```python
from build123d import *

# Parameters (mm, degrees)
F0_W     = 114.3
F0_H     = 76.2
F1_DEPTH = 3.175
F2_W     = 1.881292
F2_H     = 62.23
F3_DEPTH = 6.35


with BuildPart() as f1:
    # F0 (on Front) → F1 (new body)
    with BuildSketch(Plane.XZ):
        Rectangle(F0_W, F0_H)
    extrude(amount=-F1_DEPTH)

    # F2 (on face) → F3 (join)
    with BuildSketch(Plane.XZ):
        with Locations((-49.605354, 0)):
            Rectangle(F2_W, F2_H)
        with Locations((-38.683354, 0)):
            Rectangle(F2_W, F2_H)
        with Locations((-27.761354, 0)):
            Rectangle(F2_W, F2_H)
        with Locations((-16.839354, 0)):
            Rectangle(F2_W, F2_H)
        with Locations((-5.917354, 0)):
            Rectangle(F2_W, F2_H)
        with Locations((5.004646, 0)):
            Rectangle(F2_W, F2_H)
        with Locations((15.926646, 0)):
            Rectangle(F2_W, F2_H)
        with Locations((26.848646, 0)):
            Rectangle(F2_W, F2_H)
        with Locations((37.770646, 0)):
            Rectangle(F2_W, F2_H)
        with Locations((48.692646, 0)):
            Rectangle(F2_W, F2_H)
    extrude(amount=F3_DEPTH)


solid = f1.part
```
Geometry: final body of the model. Coordinates: model frame, mm. A direction names the side the tool comes from. Coordinates: 2 decimals unless noted, no trailing zeros. Order: outer loops, then holes, each group sorted by start corner. A loop starts at its lowest first (then second) coordinate and runs counter-clockwise, first axis right, second up. Notation, with made-up numbers: M -13.75,12 L 1.25,12 A21 ccw 1.25,45 Z; hole C -15,-11.75 d5. An arc over 180 degrees is marked long. Answer in a Markdown table with one row per item. Add a question column.
Q1. Section query B-B on x = 1. Return the cut outline in (y, z) (3 decimals), and give its area (3 significant figures).
Q2. Contact query for flat-ended pins moving along their axis: P1, Ø1.5, axis at y = -4.5, z = 6.5, coming from the -X side; P2, Ø4, axis at x = 38, y = -2.5, coming from the -Z side (3 decimals); P3, Ø1.5, axis at x = 49, y = -2.5, coming from the +Z side (3 decimals). Output: stop coordinate, or through.
Q3. Section query A-A on y = -3.75. Count the separate pieces of the cut face and the enclosed holes in it, and give its area (3 significant figures).
Q4. Line query: L1, parallel to Y at x = -11, z = -9 (3 decimals). Output: solid intervals per line, ascending.
Q5. Mould query, pull axis X, two halves, no side actions, for faces 1 (the flat face through (49.633, -3, 0)), 2 (the flat face through (-1, 2, 38.1)), 3 (the flat face through (-50.546, -3, 0)), 4 (the flat face through (-39.624, -3, 0)). Classes: released by +X, released by -X, zero draft, split by the parting line, or undercut.
Q6. Reachability of faces 5 (the flat face through (-57.15, 2, -1)), 6 (the flat face through (25.908, -3, 0)) from +Z, -Z, +X, -X, +Y, -Y: full face, straight path, thin tool, end or side. Return the list, or none.
Completed:
| question | item | result |
|---|---|---|
| 1 | outline | M 0,-38.1 L 3.175,-38.1 L 3.175,38.1 L 0,38.1 Z |
| 1 | area | 242 mm2 |
| 2 | P1 | stops at x = -50.55 |
| 2 | P2 | stops at z = -31.115 |
| 2 | P3 | stops at z = 31.115 |
| 3 | separate pieces | 10 |
| 3 | enclosed holes | 0 |
| 3 | area | 1,170 mm2 |
| 4 | L1 | y = 0 to 3.175 |
| 5 | face 1 | released by +X |
| 5 | face 2 | zero draft |
| 5 | face 3 | released by -X |
| 5 | face 4 | undercut |
| 6 | face 5 | +Z, -Z, -X, +Y, -Y |
| 6 | face 6 | +Z, -Z, -Y |
